```python
from build123d import *

# Parameters (mm, degrees)
SKETCH1_W           = 5
SKETCH1_H           = 5
BOSS_EXTRUDE1_DEPTH = 410
SKETCH1_3_W         = 5
SKETCH1_3_H         = 10
CUT_EXTRUDE1_DEPTH  = 645
CIRPATTERN1_COUNT   = 4


with BuildPart() as part:
    # Sketch1 → Boss-Extrude1 (new body)
    with BuildSketch(Plane.XY):
        Polygon((-2.5, 10), (-10, 10), (-10, -10), (10, -10), (10, 10), (2.5, 10), (2.5, 5), (-2.5, 5), align=None)
        with Locations((0, 7.5)):
            Rectangle(SKETCH1_W, SKETCH1_H)
    extrude(amount=-BOSS_EXTRUDE1_DEPTH)

    # Sketch1_3 → Cut-Extrude1 (cut)
    with BuildSketch(Plane.XY):
        with Locations((0, 10)):
            Rectangle(SKETCH1_3_W, SKETCH1_3_H)
    cut_extrude1 = extrude(amount=-CUT_EXTRUDE1_DEPTH, mode=Mode.SUBTRACT)

    # CirPattern1: Cut-Extrude1 ×4 about axis
    cirpattern1_axis = Axis((0, 0, 0), (0, 0, 1))
    for i in range(1, CIRPATTERN1_COUNT):
        add(cut_extrude1.rotate(cirpattern1_axis, i * 360 / CIRPATTERN1_COUNT), mode=Mode.SUBTRACT)


solid = part.part
```
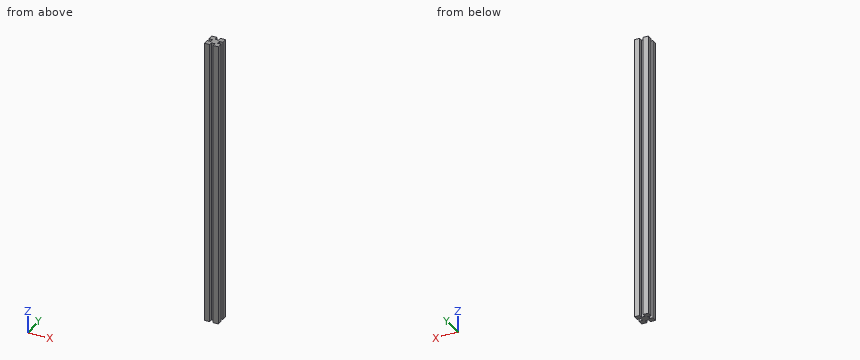
Check sheet for the modelled part. Datum: model origin and axes. Units: mm. Coordinates: 2 decimals unless noted, no trailing zeros. Order: outer loops, then holes, each group sorted by start corner. A loop starts at its lowest first (then second) coordinate and runs counter-clockwise, first axis right, second up. Notation, with made-up numbers: (24, 40.5) -> (65, 40.5) arc R14 ccw to (65, 54.5) -> close; hole circle Ø3 at (26, 25). An arc over 180 degrees is marked (long way). Write each question's results on one line, items separated by ' | '. Start each with the question number.
1) Section check A-A (z = -90). Enter the section's corners in (x, y).
2) Depth check by flat-ended pin: pin 1 (2 mm diameter, centred on y = -1, z = -51, fed in from +X); pin 2 (2.5 mm diameter, centred on y = 0.5, z = -123.5, fed in from -X); pin 3 (2 mm diameter, centred on x = -1, z = -286, fed in from +Y). Enter the tip coordinate at first touch or a pass-through.
3) Material ranges on line 1 along Y through (x, z) = (-7, -261.5); line 2 along X through (y, z) = (-0.75, -179.5), recorded low to high.
Checked values:
1) outline: (-10, -10) -> (-2.5, -10) -> (-2.5, -5) -> (2.5, -5) -> (2.5, -10) -> (10, -10) -> (10, -2.5) -> (5, -2.5) -> (5, 2.5) -> (10, 2.5) -> (10, 10) -> (2.5, 10) -> (2.5, 5) -> (-2.5, 5) -> (-2.5, 10) -> (-10, 10) -> (-10, 2.5) -> (-5, 2.5) -> (-5, -2.5) -> (-10, -2.5) -> close
2) pin 1: x = 5 | pin 2: x = -5 | pin 3: y = 5
3) line 1: -10 to -2.5, 2.5 to 10 | line 2: -5 to 5
